```python
from build123d import *

# Parameters (mm, degrees)
CYLINDER002_R     = 1.2
CYLINDER002_DEPTH = 10
ARRAY006_X_COUNT  = 2
ARRAY006_X_PITCH  = 29.6
ARRAY006_Y_COUNT  = 2
ARRAY006_Y_PITCH  = 17.8
PAD_DEPTH         = 10
ARRAY005_X_COUNT  = 2
ARRAY005_X_PITCH  = 11.8
BOX010_W          = 35.6
BOX010_H          = 23.8
BOX010_DEPTH      = 0.6
CYLINDER_R        = 1.2
CYLINDER_DEPTH    = 10
ARRAY001_X_COUNT  = 2
ARRAY001_X_PITCH  = 29.6
ARRAY001_Y_COUNT  = 2
ARRAY001_Y_PITCH  = 17.8
BOX001_W          = 6.8
BOX001_H          = 6.8
BOX001_DEPTH      = 10
ARRAY_X_COUNT     = 2
ARRAY_X_PITCH     = 11.8
BOX_W             = 35.6
BOX_H             = 23.8
BOX_DEPTH         = 2.5


with BuildPart() as bolt_hole_array003:
    # Cylinder002 → Cylinder002 (new body)
    with BuildSketch(Plane.XY):
        Circle(CYLINDER002_R)
    extrude(amount=CYLINDER002_DEPTH)

    # Array006 X: bolt hole array003 ×2


with BuildPart() as bolt_hole_array003_1:
    add(bolt_hole_array003.part)
    with Locations(*[(i * ARRAY006_X_PITCH, 0, 0) for i in range(1, ARRAY006_X_COUNT)]):
        add(bolt_hole_array003.part)

    # Array006 Y: bolt hole array003 ×2


with BuildPart() as bolt_hole_array003_2:
    add(bolt_hole_array003_1.part)
    with Locations(*[(0, i * ARRAY006_Y_PITCH, 0) for i in range(1, ARRAY006_Y_COUNT)]):
        add(bolt_hole_array003_1.part)


with BuildPart() as bolt_hole_array003_3:
    # Array006 placement: moved
    add(bolt_hole_array003_2.part.moved(Location((3, 3, 0))))


with BuildPart() as hole_fusion001:
    # Sketch001 → Pad (new body)
    with BuildSketch(Plane.XY):
        with BuildLine():
            Line((-3.4, -0.75), (-3.4, -3.4))
            Line((-3.4, -3.4), (-0.75, -3.4))
            Line((-0.75, -3.4), (-0.75, -3.197425))
            ThreePointArc((-0.352575, -2.8), (-0.633597, -2.916403), (-0.75, -3.197425))
            Line((-0.352575, -2.8), (0.352575, -2.8))
            ThreePointArc((0.75, -3.197425), (0.633597, -2.916403), (0.352575, -2.8))
            Line((0.75, -3.197425), (0.75, -3.4))
            Line((3.4, -3.4), (0.75, -3.4))
            Line((3.4, -0.75), (3.4, -3.4))
            Line((3.197425, -0.75), (3.4, -0.75))
            ThreePointArc((2.8, -0.352575), (2.916403, -0.633597), (3.197425, -0.75))
            Line((2.8, 0.352575), (2.8, -0.352575))
            ThreePointArc((3.197425, 0.75), (2.916403, 0.633597), (2.8, 0.352575))
            Line((3.4, 0.75), (3.197425, 0.75))
            Line((3.4, 3.4), (3.4, 0.75))
            Line((0.75, 3.4), (3.4, 3.4))
            Line((0.75, 3.4), (0.75, 3.197425))
            ThreePointArc((0.352575, 2.8), (0.633597, 2.916403), (0.75, 3.197425))
            Line((0.352575, 2.8), (-0.352575, 2.8))
            ThreePointArc((-0.75, 3.197425), (-0.633597, 2.916403), (-0.352575, 2.8))
            Line((-0.75, 3.197425), (-0.75, 3.4))
            Line((-3.4, 3.4), (-0.75, 3.4))
            Line((-3.4, 0.75), (-3.4, 3.4))
            Line((-3.4, 0.75), (-3.197425, 0.75))
            ThreePointArc((-2.8, 0.352575), (-2.916403, 0.633597), (-3.197425, 0.75))
            Line((-2.8, 0.352575), (-2.8, -0.352575))
            ThreePointArc((-3.197425, -0.75), (-2.916403, -0.633597), (-2.8, -0.352575))
            Line((-3.197425, -0.75), (-3.4, -0.75))
        make_face()
    extrude(amount=PAD_DEPTH)

    # Array005 X: hole fusion001 ×2


with BuildPart() as hole_fusion001_1:
    add(hole_fusion001.part)
    with Locations(*[(i * ARRAY005_X_PITCH, 0, 0) for i in range(1, ARRAY005_X_COUNT)]):
        add(hole_fusion001.part)


with BuildPart() as hole_fusion001_2:
    # Array005 placement: moved
    add(hole_fusion001_1.part.moved(Location((11.9, 11.9, 0))))

    # Fusion006: union bolt hole array003
    add(bolt_hole_array003_3.part)


with BuildPart() as obj1:
    # Box010 → Box010 (new body)
    with BuildSketch(Plane.XY):
        with Locations((17.8, 11.9)):
            Rectangle(BOX010_W, BOX010_H)
    extrude(amount=BOX010_DEPTH)

    # Cut005: cut hole fusion001
    add(hole_fusion001_2.part, mode=Mode.SUBTRACT)


with BuildPart() as obj1_1:
    # Cut005 placement: moved
    add(obj1.part.moved(Location((0, 0, 2.5))))


with BuildPart() as bolt_hole_array:
    # Cylinder → Cylinder (new body)
    with BuildSketch(Plane.XY):
        Circle(CYLINDER_R)
    extrude(amount=CYLINDER_DEPTH)

    # Array001 X: bolt hole array ×2


with BuildPart() as bolt_hole_array_1:
    add(bolt_hole_array.part)
    with Locations(*[(i * ARRAY001_X_PITCH, 0, 0) for i in range(1, ARRAY001_X_COUNT)]):
        add(bolt_hole_array.part)

    # Array001 Y: bolt hole array ×2


with BuildPart() as bolt_hole_array_2:
    add(bolt_hole_array_1.part)
    with Locations(*[(0, i * ARRAY001_Y_PITCH, 0) for i in range(1, ARRAY001_Y_COUNT)]):
        add(bolt_hole_array_1.part)


with BuildPart() as bolt_hole_array_3:
    # Array001 placement: moved
    add(bolt_hole_array_2.part.moved(Location((3, 3, 0))))


with BuildPart() as hole_fusion:
    # Box001 → Box001 (new body)
    with BuildSketch(Plane.XY):
        with Locations((3.4, 3.4)):
            Rectangle(BOX001_W, BOX001_H)
    extrude(amount=BOX001_DEPTH)

    # Array X: hole fusion ×2


with BuildPart() as hole_fusion_1:
    add(hole_fusion.part)
    with Locations(*[(i * ARRAY_X_PITCH, 0, 0) for i in range(1, ARRAY_X_COUNT)]):
        add(hole_fusion.part)


with BuildPart() as hole_fusion_2:
    # Array placement: moved
    add(hole_fusion_1.part.moved(Location((8.5, 8.5, 0))))

    # Fusion: union bolt hole array
    add(bolt_hole_array_3.part)


with BuildPart() as obj2:
    # Box → Box (new body)
    with BuildSketch(Plane.XY):
        with Locations((17.8, 11.9)):
            Rectangle(BOX_W, BOX_H)
    extrude(amount=BOX_DEPTH)

    # Cut: cut hole fusion
    add(hole_fusion_2.part, mode=Mode.SUBTRACT)

    # Fusion007: union obj1
    add(obj1_1.part)


solid = obj2.part
```
The listing builds one solid part. Answer for the finished solid, in the listing's coordinates (mm). A direction names the side the tool comes from. Give positions to 0.01 mm unless a question says otherwise; leave off trailing zeros. Order: outer loops, then holes, each group sorted by start corner. A loop starts at its lowest first (then second) coordinate and runs counter-clockwise, first axis right, second up. Notation, with made-up numbers: (13, 37) - (55, 37) arc R26 ccw to (55, 75) - close; hole circle Ø8 at (82, 46.25). An arc over 180 degrees is marked (long way). Answer in a Markdown table with one row per item. Add a question column.
Q1. The part is cut by section D-D (z = 0.55). Determine the outline of the cut face in (x, y).
Q2. The part is cut by section B-B (x = 32.6). Determine the outline of the cut face in (y, z).
Q3. Which of the six approach directions +Z, -Z, +X, -X, +Y, -Y give full straight-line access (tool end or side, diameter ignored) to faces 1 (the flat face through (0, 12, 2)), 2 (the flat face through (12, 15.3, 2))?
Q4. Find the intervals of material crossed by line 1 along Y through (x, z) = (3, 1.55); line 2 along X through (y, z) = (20.8, 1.9); line 3 along X through (y, z) = (11, 0.15), in increasing order. Write a range as [from, to].
Q5. The part is cut by section A-A (y = 10.5). Determine the outline of the cut face in (x, z), then the cut area to 3 significant figures.
Q6. Given P1, Ø0.5, axis at x = 12, y = 15, coming from the -Z side, flat-ended and moving along its own axis, determine where the tip first touches the part or whether it passes through.
Q7. For a pull along X with two mould halves and no side action, classify faces 3 (the flat face through (35.6, 12, 2)), 4 (the cylindrical face through (33.154, 19.735, 1.528)), 5 (the flat face through (18, 0, 2)) as released by +X, released by -X, zero draft, split by the parting line, or undercut.
Q8. The part is cut by section C-C (x = 14). Determine the outline of the cut face in (y, z).
Determined:
| question | item | result |
|---|---|---|
| 1 | outline | (0, 0) - (35.6, 0) - (35.6, 23.8) - (0, 23.8) - close; hole circle Ø2.4 at (3, 3); hole circle Ø2.4 at (3, 20.8); hole (8.5, 8.5) - (15.3, 8.5) - (15.3, 15.3) - (8.5, 15.3) - close; hole (20.3, 8.5) - (27.1, 8.5) - (27.1, 15.3) - (20.3, 15.3) - close; hole circle Ø2.4 at (32.6, 3); hole circle Ø2.4 at (32.6, 20.8) |
| 2 | outline | (0, 0) - (1.8, 0) - (1.8, 3.1) - (0, 3.1) - close; (4.2, 0) - (19.6, 0) - (19.6, 3.1) - (4.2, 3.1) - close; (22, 0) - (23.8, 0) - (23.8, 3.1) - (22, 3.1) - close |
| 3 | face 1 | +Z, -Z, -X, +Y, -Y |
| 3 | face 2 | -Z |
| 4 | line 1 | y = [0, 1.8], [4.2, 19.6], [22, 23.8] |
| 4 | line 2 | x = [0, 1.8], [4.2, 31.4], [33.8, 35.6] |
| 4 | line 3 | x = [0, 8.5], [15.3, 20.3], [27.1, 35.6] |
| 5 | outline | (0, 0) - (8.5, 0) - (8.5, 3.1) - (0, 3.1) - close; (15.3, 0) - (20.3, 0) - (20.3, 3.1) - (15.3, 3.1) - close; (27.1, 0) - (35.6, 0) - (35.6, 3.1) - (27.1, 3.1) - close |
| 5 | area | 68.2 mm² |
| 6 | P1 | stops at z = 2.5 |
| 7 | face 3 | released by +X |
| 7 | face 4 | undercut |
| 7 | face 5 | zero draft |
| 8 | outline | (0, 0) - (8.5, 0) - (8.5, 3.1) - (0, 3.1) - close; (15.3, 0) - (23.8, 0) - (23.8, 3.1) - (15.3, 3.1) - close |
